Input: part model. Units: mm. Frame: model coordinates. Face numbers are marked on the shaded views. Round coordinates to 2 decimals unless told otherwise and drop trailing zeros. Loops run counter-clockwise (first coordinate to the right, second up) from the corner with the lowest first, then second, coordinate; pieces in that order, holes last. Notation, with made-up numbers: (84, 18.5) - (98, 18.5) arc R28 ccw to (98, 36.5) - close; hole circle Ø6 at (34, 9). An arc over 180 degrees is marked (long way). Use CSV: the item, a comma, the result in double quotes. Start each with the question number.
1. Cut plane D-D (x = -56.5). Return loops of the section in (y, z).
2. Cut plane C-C (z = -37.5). Return loops of the section in (x, y).
3. Pin query (flat end, axial travel): P1, Ø4, axis at y = -15.5, z = -16.5, coming from the -X side; P2, Ø5, axis at y = -23.5, z = -6.5, coming from the +X side; P3, Ø10, axis at x = -47, z = -0.5, coming from the -Y side. Return the tip coordinate at first contact, or that it passes through.
4. Cut plane B-B (x = -6). Return loops of the section in (y, z), and give its area (3 significant figures).
5. Cut plane A-A (y = -20). Return loops of the section in (x, z), and give its area (3 significant figures).
6. Pull-direction query (Y, two-part tool) for the marked faces 1, 2, 3 and 4; classes: +Y half, -Y half, draft (parallel to the pull), parting line (faces both ways), or undercut.
7. Material intervals for probe 1 along X at (y, z) = (0.95, 56.5); probe 2 along X at (y, z) = (-8, 26.5); probe 3 along Y at (x, z) = (-5, 49), sorted ascending. Write a range as from..to.
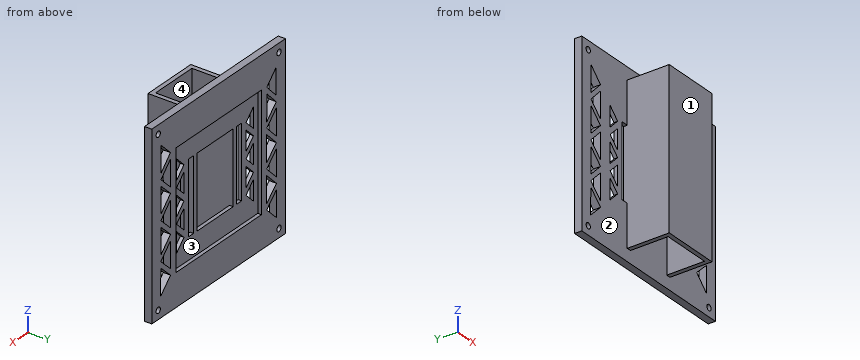
```python
from build123d import *

# Parameters (mm, degrees)
SKETCH_2_W               = 125
SKETCH_2_H               = 125
SKETCH_2_R               = 2
SKETCH_2_W_2             = 50
SKETCH_2_H_2             = 50
EXTRUDE_1_DEPTH          = 2.5
EXTRUDE_4_DEPTH          = 54
SKETCH_7_W               = 80
SKETCH_7_H               = 80
CUT_EXTRUDE_1_DEPTH      = 10
CUT_EXTRUDE_2_DEPTH      = 95.702164706
CUT_EXTRUDE_2_DEPTH_BACK = 5


with BuildPart() as part:
    # Sketch 2 → Extrude 1 (new, symmetric)
    with BuildSketch(Plane(origin=(0, 0, 0), x_dir=(1, 0, 0), z_dir=(0, 1, 0))):
        Rectangle(SKETCH_2_W, SKETCH_2_H)
        with Locations(Location((-56.5, 56.5, 0), (0, 0, 270))):
            Circle(SKETCH_2_R, mode=Mode.SUBTRACT)
        with Locations(Location((56.5, 56.5, 0), (0, 0, 270))):
            Circle(SKETCH_2_R, mode=Mode.SUBTRACT)
        with Locations(Location((-56.5, -56.5, 0), (0, 0, 270))):
            Circle(SKETCH_2_R, mode=Mode.SUBTRACT)
        with Locations(Location((56.5, -56.5, 0), (0, 0, 270))):
            Circle(SKETCH_2_R, mode=Mode.SUBTRACT)
        Rectangle(SKETCH_2_W_2, SKETCH_2_H_2, mode=Mode.SUBTRACT)
    extrude(amount=EXTRUDE_1_DEPTH, both=True)

    # Sketch 6 → Extrude 4 (add, symmetric)
    with BuildSketch(Plane.XY):
        Polygon((-20, 0), (-20, -31.5), (20, -31.5), (20, 0), (17, 0), (17, -28.5), (-17, -28.5), (-17, 0), align=None)
    extrude(amount=EXTRUDE_4_DEPTH, both=True)

    # Sketch 7 → Cut-Extrude 1 (cut)
    with BuildSketch(Plane(origin=(0, 0, 0), x_dir=(1, 0, 0), z_dir=(0, 1, 0))):
        Rectangle(SKETCH_7_W, SKETCH_7_H)
    extrude(amount=CUT_EXTRUDE_1_DEPTH, mode=Mode.SUBTRACT)

    # Sketch 8 → Cut-Extrude 2 (cut, two sides: drawn at the far end of the back side and taken through both)
    with BuildSketch(Plane(origin=(0, 2.5, 0), x_dir=(1, 0, 0), z_dir=(0, 1, 0)).offset(-CUT_EXTRUDE_2_DEPTH_BACK)):
        Polygon((54.07931581, 22.285580831), (54.015526938, 4.28569386), (44.986382589, 13.073341514), align=None)
        Polygon((36, -30.343145751), (36, -16.343145751), (29, -23.343145751), align=None)
        Polygon((29, 18.671572875), (29, 4.671572875), (36, 11.671572875), align=None)
        Polygon((36, 30.343145751), (29, 23.343145751), (36, 16.343145751), align=None)
        Polygon((53.829622097, -48.172767848), (45.041121619, -39.384267369), (53.893419828, -30.170381277), align=None)
        Polygon((45.036831341, -35.272800588), (45.018048518, -17.272810388), (53.90806007, -26.039210725), align=None)
        Polygon((44.95901306, 39.30215881), (54.172270373, 48.515416123), (54.1084815, 30.515529152), align=None)
        Polygon((53.922585518, -21.940432956), (45.013752114, -13.155472476), (53.986361248, -3.944254461), align=None)
        Polygon((45.009460593, -9.042814869), (54.001004771, 0.18784173), (44.99067777, 8.957175331), align=None)
        Polygon((44.982089846, 17.187170851), (54.093962598, 26.418598199), (44.963307022, 35.187161051), align=None)
        Polygon((29, 0), (36, 7), (36, -7), align=None)
        Polygon((36, -11.671572875), (29, -4.671572875), (29, -18.671572875), align=None)
        Polygon((-36, -7), (-36, 7), (-29, 0), align=None)
        Polygon((-29, -4.671572875), (-29, -18.671572875), (-36, -11.671572875), align=None)
        Polygon((-36, 16.343145751), (-36, 30.343145751), (-29, 23.343145751), align=None)
        Polygon((-36, -16.343145751), (-29, -23.343145751), (-36, -30.343145751), align=None)
        Polygon((-36, 11.671572875), (-29, 4.671572875), (-29, 18.671572875), align=None)
        Polygon((-53.893419828, -30.170381277), (-53.829622097, -48.172767848), (-45.041121619, -39.384267369), align=None)
        Polygon((-45.009460593, -9.042814869), (-44.99067777, 8.957175331), (-54.001004771, 0.18784173), align=None)
        Polygon((-53.986361248, -3.944254461), (-53.922585518, -21.940432956), (-45.013752114, -13.155472476), align=None)
        Polygon((-44.982089846, 17.187170851), (-44.963307022, 35.187161051), (-54.093962598, 26.418598199), align=None)
        Polygon((-54.1084815, 30.515529152), (-44.95901306, 39.30215881), (-54.172270373, 48.515416123), align=None)
        Polygon((-44.986382589, 13.073341514), (-54.07931581, 22.285580831), (-54.015526938, 4.28569386), align=None)
        Polygon((-53.90806007, -26.039210725), (-45.018048518, -17.272810388), (-45.036831341, -35.272800588), align=None)
    extrude(amount=CUT_EXTRUDE_2_DEPTH + CUT_EXTRUDE_2_DEPTH_BACK, mode=Mode.SUBTRACT)


solid = part.part
```
Established:
1,outline,"(-2.5, -62.5) - (2.5, -62.5) - (2.5, -58.5) - (-2.5, -58.5) - close; (-2.5, -54.5) - (2.5, -54.5) - (2.5, 54.5) - (-2.5, 54.5) - close; (-2.5, 58.5) - (2.5, 58.5) - (2.5, 62.5) - (-2.5, 62.5) - close"
2,outline,"(-62.5, -2.5) - (-54.13, -2.5) - (-54.13, 2.5) - (-62.5, 2.5) - close; (-46.84, -2.5) - (-20, -2.5) - (-20, -31.5) - (20, -31.5) - (20, -2.5) - (46.84, -2.5) - (46.84, 2.5) - (40, 2.5) - (40, 0) - (-40, 0) - (-40, 2.5) - (-46.84, 2.5) - close; (54.13, -2.5) - (62.5, -2.5) - (62.5, 2.5) - (54.13, 2.5) - close; hole (-17, -28.5) - (17, -28.5) - (17, -2.5) - (-17, -2.5) - close"
3,P1,"stops at x = -20"
3,P2,"stops at x = 20"
3,P3,"stops at y = -2.5"
4,outline,"(-31.5, -54) - (-28.5, -54) - (-28.5, 54) - (-31.5, 54) - close; (-2.5, -62.5) - (2.5, -62.5) - (2.5, -40) - (0, -40) - (0, -25) - (-2.5, -25) - close; (-2.5, 25) - (0, 25) - (0, 40) - (2.5, 40) - (2.5, 62.5) - (-2.5, 62.5) - close"
4,area,"624 mm2"
5,outline,"(-20, -54) - (-17, -54) - (-17, 54) - (-20, 54) - close; (17, -54) - (20, -54) - (20, 54) - (17, 54) - close"
5,area,"648 mm2"
6,face 1,"-Y half"
6,face 2,"undercut"
6,face 3,"+Y half"
6,face 4,"undercut"
7,probe 1,"x = -62.5..-58.5, -54.5..54.5, 58.5..62.5"
7,probe 2,"x = -20..-17, 17..20"
7,probe 3,"y = -31.5..-28.5, -2.5..2.5"
